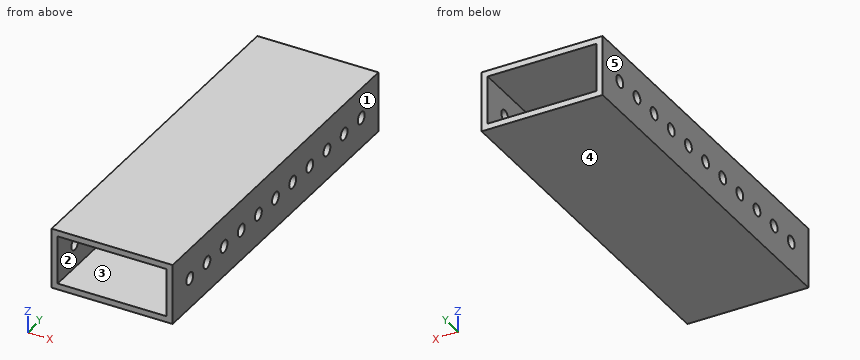
```python
from build123d import *

# Parameters (mm, degrees)
SKETCH1_W           = 50.8
SKETCH1_H           = 25.4
SKETCH1_W_2         = 45.72
SKETCH1_H_2         = 20.32
BOSS_EXTRUDE2_DEPTH = 152.4
SKETCH2_R           = 2.54
CUT_EXTRUDE1_DEPTH  = 127


with BuildPart() as part:
    # Sketch1 → Boss-Extrude2 (new body)
    with BuildSketch(Plane(origin=(0, 0, 0), x_dir=(1, 0, 0), z_dir=(0, 1, 0))):
        with Locations((-34.550728477, 5.021125828)):
            Rectangle(SKETCH1_W, SKETCH1_H)
        with Locations((-34.550728477, 5.021125828)):
            Rectangle(SKETCH1_W_2, SKETCH1_H_2, mode=Mode.SUBTRACT)
    extrude(amount=BOSS_EXTRUDE2_DEPTH)

    # Sketch2 → Cut-Extrude1 (cut)
    with BuildSketch(Plane(origin=(-9.150728477, 0, 0), x_dir=(0, 0, -1), z_dir=(1, 0, 0))):
        with Locations((5.021125828, 139.7)):
            Circle(SKETCH2_R)
        with Locations((5.021125828, 127)):
            Circle(SKETCH2_R)
        with Locations((5.021125828, 114.3)):
            Circle(SKETCH2_R)
        with Locations((5.021125828, 101.6)):
            Circle(SKETCH2_R)
        with Locations((5.021125828, 88.9)):
            Circle(SKETCH2_R)
        with Locations((5.021125828, 76.2)):
            Circle(SKETCH2_R)
        with Locations((5.021125828, 63.5)):
            Circle(SKETCH2_R)
        with Locations((5.021125828, 50.8)):
            Circle(SKETCH2_R)
        with Locations((5.021125828, 38.1)):
            Circle(SKETCH2_R)
        with Locations((5.021125828, 25.4)):
            Circle(SKETCH2_R)
        with Locations((5.021125828, 12.7)):
            Circle(SKETCH2_R)
    extrude(amount=-CUT_EXTRUDE1_DEPTH, mode=Mode.SUBTRACT)


solid = part.part
```
Can you work these out from the model? Positions are in its coordinate system, mm. Face numbers are marked on the shaded views. A direction names the side the tool comes from. Give positions to 0.01 mm unless a question says otherwise; leave off trailing zeros. Loops run counter-clockwise (first coordinate to the right, second up) from the corner with the lowest first, then second, coordinate; pieces in that order, holes last. Notation, with made-up numbers: M -21.75,63 L -6.75,63 A19 ccw -6.75,88 Z; hole C 45,72 d8. An arc over 180 degrees is marked long. Use one line per item in the form item = value. Start each with the question number.
(1) I want a section at B-B, the plane y = 25.4. Write out the boundary of the cut face in (x, z), and give its area (3 significant figures).
(2) I want a section at A-A, the plane x = -52.5. Write out the boundary of the cut face in (y, z), and give its area (3 significant figures).
(3) On a 3-axis mill with a long thin cutter (end or side, diameter ignored), from which of +Z, -Z, +X, -X, +Y, -Y can I reach the whole of each face in a straight line? I mean the marked faces 1 and 2. Say none if no direction works.
(4) Thinking about a two-plate mould opening in Z: for the marked faces 3, 4 and 5, which applies, released by +Z, released by -Z, zero draft, split by the parting line, or undercut?
(5) Please list where these lines run through material, in increasing order: line 1 (Z direction, x = -23.5, y = 102); line 2 (X direction, y = 99, z = -8.5); line 3 (Z direction, x = -58, y = 113).
(6) I want a section at D-D, the plane z = -4.5. State how many separate pieces and enclosed holes the cut face has, and give its area (3 significant figures).
(7) I want a section at C-C, the plane z = -10.25. Write out the boundary of the cut face in (x, y), and give its area (3 significant figures).
Worked out:
q1.outline = M -59.95,-17.72 L -9.15,-17.72 L -9.15,-7.56 L -11.69,-7.56 L -11.69,-15.18 L -57.41,-15.18 L -57.41,-7.56 L -59.95,-7.56 Z; M -59.95,-2.48 L -57.41,-2.48 L -57.41,5.14 L -11.69,5.14 L -11.69,-2.48 L -9.15,-2.48 L -9.15,7.68 L -59.95,7.68 Z
q1.area = 335 mm²
q2.outline = M 0,-17.72 L 152.4,-17.72 L 152.4,-15.18 L 0,-15.18 Z; M 0,5.14 L 152.4,5.14 L 152.4,7.68 L 0,7.68 Z
q2.area = 774 mm²
q3.face_1 = +Z, -Z, +X, +Y, -Y
q3.face_2 = +Y, -Y
q4.face_3 = undercut
q4.face_4 = released by -Z
q4.face_5 = zero draft
q5.line_1 = -17.72 to -15.18, 5.14 to 7.68
q5.line_2 = -59.95 to -57.41, -11.69 to -9.15
q5.line_3 = -17.72 to -7.2, -2.84 to 7.68
q6.separate_pieces = 24
q6.enclosed_holes = 0
q6.area = 496 mm²
q7.outline = M -59.95,0 L -57.41,0 L -57.41,152.4 L -59.95,152.4 Z; M -11.69,0 L -9.15,0 L -9.15,152.4 L -11.69,152.4 Z
q7.area = 774 mm²
